For this review, take the finished solid that the model builds, in its own axes (mm). A direction names the side the tool comes from. Coordinates: 2 decimals unless noted, no trailing zeros. Loops run counter-clockwise (first coordinate to the right, second up) from the corner with the lowest first, then second, coordinate; pieces in that order, holes last. Notation, with made-up numbers: (54, -5.75) -> (81, -5.75) arc R26 ccw to (81, 13.25) -> close; hole circle Ø7 at (66.25, 74.5). An arc over 180 degrees is marked (long way). Use a Markdown table: item, result.
from build123d import *

# Parameters (mm, degrees)
BOSS_EXTRUDE1_DEPTH = 44
SKETCH3_R           = 1.5
CUT_EXTRUDE1_DEPTH  = 30
SKETCH4_R           = 1.5
CUT_EXTRUDE2_DEPTH  = 30


with BuildPart() as part:
    # Sketch2 → Boss-Extrude1 (new body)
    with BuildSketch(Plane.XY):
        Polygon((24.8, 15), (26.8, 15), (26.8, 0), (0, 0), (0, 15), (2, 15), (2, 2), (24.8, 2), align=None)
    extrude(amount=BOSS_EXTRUDE1_DEPTH)

    # Sketch3 → Cut-Extrude1 (cut)
    with BuildSketch(Plane.XZ):
        with Locations(Location((21.4, 36, 0), (0, 0, 270))):
            Circle(SKETCH3_R)
        with Locations(Location((13.4, 8, 0), (0, 0, 270))):
            Circle(SKETCH3_R)
        with Locations(Location((5.4, 36, 0), (0, 0, 270))):
            Circle(SKETCH3_R)
        with BuildLine():
            Line((22.4, 17.75), (4.4, 17.75))
            ThreePointArc((4.4, 17.75), (2.15, 20), (4.4, 22.25))
            Line((4.4, 22.25), (22.4, 22.25))
            ThreePointArc((22.4, 22.25), (24.65, 20), (22.4, 17.75))
        make_face()
    extrude(amount=-CUT_EXTRUDE1_DEPTH, mode=Mode.SUBTRACT)

    # Sketch4 → Cut-Extrude2 (cut)
    with BuildSketch(Plane.ZY):
        with Locations((6, 11)):
            Circle(SKETCH4_R)
        with Locations((38, 11)):
            Circle(SKETCH4_R)
    extrude(amount=-CUT_EXTRUDE2_DEPTH, mode=Mode.SUBTRACT)


solid = part.part
(1) Take a section at D-D on z = 40.5. Write out the cut boundary in (x, y), plus the area to 3 significant figures.
Found:
| item | result |
|---|---|
| outline | (0, 0) -> (26.8, 0) -> (26.8, 15) -> (24.8, 15) -> (24.8, 2) -> (2, 2) -> (2, 15) -> (0, 15) -> close |
| area | 106 mm^2 |
(2) Take a section at B-B on z = 8. Write out the cut boundary in (x, y).
Found:
| item | result |
|---|---|
| outline | (0, 0) -> (11.9, 0) -> (11.9, 2) -> (2, 2) -> (2, 15) -> (0, 15) -> close; (14.9, 0) -> (26.8, 0) -> (26.8, 15) -> (24.8, 15) -> (24.8, 2) -> (14.9, 2) -> close |
(3) For faces 1 (the face through (24.8, 8, 22)), 2 (the face through (25.8, 10.1, 36.8)), 3 (the face through (2.15, 0.99, 19.95)), list the 3-axis set-ups (+Z, -Z, +X, -X, +Y, -Y) from which the entire face can be reached by the end or side of a thin tool; tool diameter is ignored.
Found:
| item | result |
|---|---|
| face 1 | +Z, -Z, +Y |
| face 2 | +X, -X |
| face 3 | +Y, -Y |
(4) Take a section at C-C on y = 3.75. Write out the cut boundary in (x, z), plus the area to 3 significant figures.
Found:
| item | result |
|---|---|
| outline | (0, 0) -> (2, 0) -> (2, 44) -> (0, 44) -> close; (24.8, 0) -> (26.8, 0) -> (26.8, 44) -> (24.8, 44) -> close |
| area | 176 mm^2 |
(5) Take a section at A-A on x = 5.4. Write out the cut boundary in (y, z).
Found:
| item | result |
|---|---|
| outline | (0, 0) -> (2, 0) -> (2, 17.75) -> (0, 17.75) -> close; (0, 22.25) -> (2, 22.25) -> (2, 34.5) -> (0, 34.5) -> close; (0, 37.5) -> (2, 37.5) -> (2, 44) -> (0, 44) -> close |
(6) For line 1 along X through (y, z) = (0.6, 8); line 2 along X through (y, z) = (5.25, 40.5); line 3 along Y through (x, z) = (25.95, 38), list the stretches that pass through material, from the lowest coordinate up.
Found:
| item | result |
|---|---|
| line 1 | x = 0 to 11.9, 14.9 to 26.8 |
| line 2 | x = 0 to 2, 24.8 to 26.8 |
| line 3 | y = 0 to 9.5, 12.5 to 15 |
(7) Mouldability with a two-part tool opening along X and no side actions: class faces 4 (the face through (0, 7, 22)), 5 (the face through (13, 1, 0)), 6 (the face through (20.5, 1, 37.2)), 7 (the face through (24.65, 0.99, 20.05)) as pulls with the +X half, pulls with the -X half, needs draft (parallel to the pull), parting line crosses it, or undercut.
Found:
| item | result |
|---|---|
| face 4 | pulls with the -X half |
| face 5 | needs draft |
| face 6 | undercut |
| face 7 | undercut |
(8) For pin 1 Ø2.5 at (x, z) = (5.4, 36) entering from -Y; pin 2 Ø6 at (x, z) = (19.5, 22) entering from +Y, all flat-tipped, find the tip position at first contact; note any pin that passes through.
Found:
| item | result |
|---|---|
| pin 1 | passes through |
| pin 2 | stops at y = 2 |
